```python
from build123d import *

# Parameters (mm, degrees)
SKETCH1_W                                         = 35
SKETCH1_H                                         = 30
BOSS_EXTRUDE1_DEPTH                               = 20
SHELL1_T                                          = -1
SKETCH6_R                                         = 2
BOSS_EXTRUDE5_DEPTH                               = 5
CSK_FOR_0_FLAT_HEAD_MACHINE_SCREW_100_D           = 1.778
CSK_FOR_0_FLAT_HEAD_MACHINE_SCREW_100_CSINK_D     = 3.0226
CSK_FOR_0_FLAT_HEAD_MACHINE_SCREW_100_CSINK_ANGLE = 100
SKETCH11_R                                        = 1.5
BOSS_EXTRUDE6_DEPTH                               = 19.5
CSK_FOR_0_FLAT_HEAD_MACHINE_SCREW_2_D             = 1.778
CSK_FOR_0_FLAT_HEAD_MACHINE_SCREW_2_CSINK_D       = 3.0226
CSK_FOR_0_FLAT_HEAD_MACHINE_SCREW_2_CSINK_ANGLE   = 100
SKETCH16_W                                        = 15.652105204
SKETCH16_H                                        = 5
CUT_EXTRUDE1_DEPTH                                = 7.5
FILLET1_R                                         = 3
FILLET2_R                                         = 3


with BuildPart() as part:
    # Sketch1 → Boss-Extrude1 (new body)
    with BuildSketch(Plane.XY):
        with Locations((17.5, 15)):
            Rectangle(SKETCH1_W, SKETCH1_H)
    extrude(amount=BOSS_EXTRUDE1_DEPTH)

    # Shell1
    shell1_openings = [part.faces().sort_by_distance(p)[0] for p in [
        (17.5, 15, 20),
    ]]
    offset(amount=SHELL1_T, openings=shell1_openings, kind=Kind.INTERSECTION)

    # Sketch6 → Boss-Extrude5 (add)
    with BuildSketch(Plane.XY.offset(1)):
        with Locations(Location((31, 4, 0), (0, 0, 180))):
            Circle(SKETCH6_R)
        with Locations(Location((6, 4, 0), (0, 0, 180))):
            Circle(SKETCH6_R)
    extrude(amount=BOSS_EXTRUDE5_DEPTH)

    # CSK for _0 Flat Head Machine Screw _100 (through all)
    with Locations(Plane.XY.offset(6)):
        with Locations((5.574399883, 3.50151513), (31, 4)):
            CounterSinkHole(CSK_FOR_0_FLAT_HEAD_MACHINE_SCREW_100_D / 2, CSK_FOR_0_FLAT_HEAD_MACHINE_SCREW_100_CSINK_D / 2, counter_sink_angle=CSK_FOR_0_FLAT_HEAD_MACHINE_SCREW_100_CSINK_ANGLE)

    # Sketch11 → Boss-Extrude6 (add)
    with BuildSketch(Plane.XY.offset(1)):
        with Locations(Location((3, 27, 0), (0, 0, 180))):
            Circle(SKETCH11_R)
        with Locations(Location((32, 27, 0), (0, 0, 180))):
            Circle(SKETCH11_R)
    extrude(amount=BOSS_EXTRUDE6_DEPTH)

    # CSK for _0 Flat Head Machine Screw _ 2 (through all)
    with Locations(Plane.XY.offset(20.5)):
        with Locations((31.925463408, 26.981922801), (3, 27)):
            CounterSinkHole(CSK_FOR_0_FLAT_HEAD_MACHINE_SCREW_2_D / 2, CSK_FOR_0_FLAT_HEAD_MACHINE_SCREW_2_CSINK_D / 2, counter_sink_angle=CSK_FOR_0_FLAT_HEAD_MACHINE_SCREW_2_CSINK_ANGLE)

    # Sketch16 → Cut-Extrude1 (cut)
    with BuildSketch(Plane(origin=(0, 30, 0), x_dir=(1, 0, 0), z_dir=(0, 1, 0))):
        with Locations((17.173947398, -10.424136078)):
            Rectangle(SKETCH16_W, SKETCH16_H)
    extrude(amount=-CUT_EXTRUDE1_DEPTH, mode=Mode.SUBTRACT)

    # Fillet1
    # the kernel refuses this fillet: 3 mm, written as the material it adds along each edge
    with BuildSketch(Plane(origin=(3, 27, 1), x_dir=(-1, 0, 0), z_dir=(0, 1, 0))) as fillet1_piece_1_section:
        with BuildLine():
            CenterArc((1.5 + FILLET1_R, FILLET1_R), FILLET1_R, 180, 90)
            Line((1.5, FILLET1_R), (1.5, 0))
            Line((1.5, 0), (1.5 + FILLET1_R, 0))
        make_face()
    fillet1_piece_1 = revolve(axis=Axis((3, 27, 1), (0, 0, 1)), mode=Mode.PRIVATE)
    fillet1_piece_1 = split(fillet1_piece_1, bisect_by=Plane(origin=(1, 27, 1.859549256), z_dir=(1, 0, 0)), keep=Keep.TOP, mode=Mode.PRIVATE)
    fillet1_piece_1 = split(fillet1_piece_1, bisect_by=Plane(origin=(5.359549256, 29, 1.859549256), z_dir=(0, -1, 0)), keep=Keep.TOP, mode=Mode.PRIVATE)
    add(fillet1_piece_1)
    with BuildSketch(Plane(origin=(32, 27, 1), x_dir=(-1, 0, 0), z_dir=(0, 1, 0))) as fillet1_piece_2_section:
        with BuildLine():
            CenterArc((1.5 + FILLET1_R, FILLET1_R), FILLET1_R, 180, 90)
            Line((1.5, FILLET1_R), (1.5, 0))
            Line((1.5, 0), (1.5 + FILLET1_R, 0))
        make_face()
    fillet1_piece_2 = revolve(axis=Axis((32, 27, 1), (0, 0, 1)), mode=Mode.PRIVATE)
    fillet1_piece_2 = split(fillet1_piece_2, bisect_by=Plane(origin=(30.141729678, 29, 1.076089877), z_dir=(0, -1, 0)), keep=Keep.TOP, mode=Mode.PRIVATE)
    fillet1_piece_2 = split(fillet1_piece_2, bisect_by=Plane(origin=(34, 23.781381388, 1.076089877), z_dir=(-1, 0, 0)), keep=Keep.TOP, mode=Mode.PRIVATE)
    add(fillet1_piece_2)

    # Fillet2
    # the kernel refuses this fillet: 3 mm, written as the material it adds along each edge
    with BuildSketch(Plane(origin=(31, 4, 1), x_dir=(-1, 0, 0), z_dir=(0, 1, 0))) as fillet2_piece_1_section:
        with BuildLine():
            CenterArc((2 + FILLET2_R, FILLET2_R), FILLET2_R, 180, 90)
            Line((2, FILLET2_R), (2, 0))
            Line((2, 0), (2 + FILLET2_R, 0))
        make_face()
    fillet2_piece_1 = revolve(axis=Axis((31, 4, 1), (0, 0, 1)), mode=Mode.PRIVATE)
    fillet2_piece_1 = split(fillet2_piece_1, bisect_by=Plane(origin=(33.856939256, 0, 1.856939256), z_dir=(0, 1, 0)), keep=Keep.TOP, mode=Mode.PRIVATE)
    fillet2_piece_1 = split(fillet2_piece_1, bisect_by=Plane(origin=(35, 4, 1.856939256), z_dir=(-1, 0, 0)), keep=Keep.TOP, mode=Mode.PRIVATE)
    add(fillet2_piece_1)
    with BuildSketch(Plane(origin=(6, 4, 1), x_dir=(-1, 0, 0), z_dir=(0, 1, 0))) as fillet2_piece_2_section:
        with BuildLine():
            CenterArc((2 + FILLET2_R, FILLET2_R), FILLET2_R, 180, 90)
            Line((2, FILLET2_R), (2, 0))
            Line((2, 0), (2 + FILLET2_R, 0))
        make_face()
    fillet2_piece_2 = revolve(axis=Axis((6, 4, 1), (0, 0, 1)), mode=Mode.PRIVATE)
    fillet2_piece_2 = split(fillet2_piece_2, bisect_by=Plane(origin=(8.856531723, 0, 1.856531723), z_dir=(0, 1, 0)), keep=Keep.TOP, mode=Mode.PRIVATE)
    add(fillet2_piece_2)


solid = part.part
```
Build history of the part. All positions in model axes, mm. A direction names the side the tool comes from. Round coordinates to 2 decimals unless told otherwise and drop trailing zeros. Order: outer loops, then holes, each group sorted by start corner. A loop starts at its lowest first (then second) coordinate and runs counter-clockwise, first axis right, second up. Notation, with made-up numbers: (-15.75, 68.5) -> (-10.75, 68.5) arc R25 cw to (-10.75, 84.5) -> close; hole circle Ø1 at (2, -3). An arc over 180 degrees is marked (long way). Answer in a Markdown table with one row per item.
1) Band-saw the part on A-A on x = 13. Give the cut face in (y, z), and give its area (3 significant figures).
Values:
| item | result |
|---|---|
| outline | (0, 0) -> (30, 0) -> (30, 7.92) -> (29, 7.92) -> (29, 1) -> (1, 1) -> (1, 20) -> (0, 20) -> close; (29, 12.92) -> (30, 12.92) -> (30, 20) -> (29, 20) -> close |
| area | 63.0 mm2 |
2) Wall check: L1, parallel to X at y = 27, z = 10; L2, parallel to Y at x = 3, z = 14.5; L3, parallel to Y at x = 9, z = 14. Give the ranges that are in metal, low to high.
Values:
| item | result |
|---|---|
| L1 | 0 to 1, 1.5 to 2.11, 3.89 to 4.5, 30.5 to 31.04, 32.81 to 33.5, 34 to 35 |
| L2 | 0 to 1, 25.5 to 26.11, 27.89 to 28.5, 29 to 30 |
| L3 | 0 to 1, 29 to 30 |
3) Pin check, flat tips, straight feed: P1, Ø1.1, axis at x = 1.5, y = 2, coming from the +Z side; P2, Ø1.4, axis at x = 3, y = 27, coming from the -Z side; P3, Ø2, axis at x = 31, y = 4, coming from the +Z side; P4, Ø8.5, axis at x = 21.5, y = 12, coming from the +Z side. Stop position of each tip, or through.
Values:
| item | result |
|---|---|
| P1 | z = 20 |
| P2 | through |
| P3 | z = 5.57 |
| P4 | z = 1 |
4) Mould opens along Y. For faces 4 (the flat face through (17.3, 30, 7.6)), 5 (the cylindrical face through (6.28, 2.96, 2.7)), 6 (the flat face through (0, 15, 10)) say: released by +Y, released by -Y, zero draft, split by the parting line, or undercut.
Values:
| item | result |
|---|---|
| face 4 | released by +Y |
| face 5 | undercut |
| face 6 | zero draft |
5) Band-saw the part on C-C on y = 14.5. Give the cut face in (x, z), and give its area (3 significant figures).
Values:
| item | result |
|---|---|
| outline | (0, 0) -> (35, 0) -> (35, 20) -> (34, 20) -> (34, 1) -> (1, 1) -> (1, 20) -> (0, 20) -> close |
| area | 73.0 mm2 |
6) Which spindle directions (+Z, -Z, +X, -X, +Y, -Y) get a long thin tool onto all of the face, cutting with end or side? Do faces 1 (the flat face through (17, 0, 10)), 2 (the flat face through (17.1, 29.5, 12.924)), 3 (the flat face through (7, 5, 6)). Say none if no direction does.
Values:
| item | result |
|---|---|
| face 1 | +Z, -Z, +X, -X, -Y |
| face 2 | +Y |
| face 3 | +Z |
7) Band-saw the part on B-B on z = 16. Give the cut face in (x, y), and give its area (3 significant figures).
Values:
| item | result |
|---|---|
| outline | (0, 0) -> (35, 0) -> (35, 30) -> (0, 30) -> close; circle Ø3 at (3, 27); circle Ø3 at (32, 27); hole (1, 1) -> (34, 1) -> (34, 29) -> (1, 29) -> close; hole circle Ø1.78 at (3, 27); hole circle Ø1.78 at (31.93, 26.98) |
| area | 135 mm2 |
8) Band-saw the part on D-D on z = 10.25. Give the cut face in (x, y), and give its area (3 significant figures).
Values:
| item | result |
|---|---|
| outline | (0, 0) -> (35, 0) -> (35, 30) -> (25, 30) -> (25, 29) -> (34, 29) -> (34, 1) -> (1, 1) -> (1, 29) -> (9.35, 29) -> (9.35, 30) -> (0, 30) -> close; circle Ø3 at (3, 27); circle Ø3 at (32, 27); hole circle Ø1.78 at (3, 27); hole circle Ø1.78 at (31.93, 26.98) |
| area | 120 mm2 |
